from build123d import *

# Parameters (mm, degrees)
SKETCH1_R                = 1.75
BOSS_EXTRUDE1_DEPTH      = 23
FILLET3_R                = 10
BOSS_EXTRUDE2_DEPTH      = 4.5
BOSS_EXTRUDE2_DEPTH_BACK = 4
SKETCH3_R                = 1.75
SKETCH4_R                = 11.25
CUT_EXTRUDE1_DEPTH       = 7
SKETCH5_R                = 13
CUT_EXTRUDE2_DEPTH       = 1.5
SKETCH6_R                = 3
CUT_EXTRUDE3_DEPTH       = 12
CUT_EXTRUDE4_DEPTH       = 1
FILLET7_R                = 3
FILLET8_R                = 10


with BuildPart() as part:
    # Sketch1 → Boss-Extrude1 (new body)
    with BuildSketch(Plane.XY):
        with BuildLine():
            Line((-8.845360825, 11.520618557), (-14.845360825, 2.520618557))
            Line((-14.845360825, 2.520618557), (-14.845360825, -0.479381443))
            Line((-14.845360825, -0.479381443), (-9.845360825, -0.479381443))
            Line((-9.845360825, -0.479381443), (-8.845360825, 0.520618557))
            ThreePointArc((-8.845360825, 0.520618557), (-1.696742799, 7.320595709), (6.83903909, 12.26861112))
            Line((6.83903909, 12.26861112), (9.318301605, 19.26861112))
            ThreePointArc((9.318301605, 19.26861112), (-0.918731235, 18.102760488), (-8.845360825, 11.520618557))
        make_face()
        with Locations((-8.845360825, 5.020618557)):
            Circle(SKETCH1_R, mode=Mode.SUBTRACT)
        with Locations((3.154639175, 15.020618557)):
            Circle(SKETCH1_R, mode=Mode.SUBTRACT)
    extrude(amount=BOSS_EXTRUDE1_DEPTH)

    # Fillet3
    # the kernel refuses this fillet: 10 mm, written as the material it takes off along each edge
    with BuildSketch(Plane(origin=(-9.845360825, -0.479381443, -10.932362995), x_dir=(-1, 0, 0), z_dir=(0, 0, 1))) as fillet3_piece_1:
        with BuildLine():
            CenterArc((4.372945198, -10), FILLET3_R, 90, 46.455884642)
            Line((-2.87549632, -3.110871204), (-3.600340471, -2.421958325))
            ThreePointArc((-3.600340471, -2.421958325), (-1.769425443, -0.361263367), (-0.707106781, 0.707106781))
            Line((-0.707106781, 0.707106781), (0, 1))
            Line((0, 1), (4.372945198, 1))
            Line((4.372945198, 1), (4.372945198, 0))
        make_face()
    extrude(amount=44.86472599, mode=Mode.SUBTRACT)

    # Sketch3 → Boss-Extrude2 (add, two sides: drawn at the far end of the back side and taken through both)
    with BuildSketch(Plane.XY.offset(23).offset(-BOSS_EXTRUDE2_DEPTH_BACK)):
        with BuildLine():
            Line((-14.845360825, 2.520618557), (-14.845360825, -0.479381443))
            Line((-14.845360825, -0.479381443), (-12.565000182, -16.009144975))
            ThreePointArc((-12.565000182, -16.009144975), (8.709502938, -29.945300767), (20.013420995, -7.162799635))
            Line((20.013420995, -7.162799635), (9.318301605, 19.26861112))
            ThreePointArc((9.318301605, 19.26861112), (-0.918731235, 18.102760488), (-8.845360825, 11.520618557))
            Line((-8.845360825, 11.520618557), (-14.845360825, 2.520618557))
        make_face()
        with Locations((3.154639175, 15.020618557)):
            Circle(SKETCH3_R, mode=Mode.SUBTRACT)
        with Locations((-8.845360825, 5.020618557)):
            Circle(SKETCH3_R, mode=Mode.SUBTRACT)
    extrude(amount=BOSS_EXTRUDE2_DEPTH + BOSS_EXTRUDE2_DEPTH_BACK)

    # Sketch4 → Cut-Extrude1 (cut)
    with BuildSketch(Plane(origin=(0, 0, 19), x_dir=(-1, 0, 0), z_dir=(0, 0, -1))):
        with Locations((-4.254639175, -13.539381443)):
            Circle(SKETCH4_R)
    extrude(amount=-CUT_EXTRUDE1_DEPTH, mode=Mode.SUBTRACT)

    # Sketch5 → Cut-Extrude2 (cut)
    with BuildSketch(Plane(origin=(0, 0, 19), x_dir=(-1, 0, 0), z_dir=(0, 0, -1))):
        with Locations((-4.254639175, -13.539381443)):
            Circle(SKETCH5_R)
    extrude(amount=-CUT_EXTRUDE2_DEPTH, mode=Mode.SUBTRACT)

    # Sketch6 → Cut-Extrude3 (cut)
    with BuildSketch(Plane.XY.offset(27.5)):
        with Locations((-8.845360825, 5.020618557)):
            Circle(SKETCH6_R)
        with Locations((3.154639175, 15.020618557)):
            Circle(SKETCH6_R)
    extrude(amount=-CUT_EXTRUDE3_DEPTH, mode=Mode.SUBTRACT)

    # Sketch7 → Cut-Extrude4 (cut)
    with BuildSketch(Plane(origin=(0, 0, 19), x_dir=(-1, 0, 0), z_dir=(0, 0, -1))):
        with BuildLine():
            Line((-19.320512006, -15.73138888), (-26.521187379, 19.26861112))
            Line((-26.521187379, 19.26861112), (-9.318301605, 19.26861112))
            Line((-9.318301605, 19.26861112), (-6.83903909, 12.26861112))
            ThreePointArc((-6.83903909, 12.26861112), (0.552528201, 8.148031782), (6.969864505, 2.631489761))
            Line((6.969864505, 2.631489761), (-2.943055137, 1.26861112))
            ThreePointArc((-2.943055137, 1.26861112), (-15.267616881, -3.247010549), (-19.320512006, -15.73138888))
        make_face()
    extrude(amount=-CUT_EXTRUDE4_DEPTH, mode=Mode.SUBTRACT)

    # Fillet7
    # the kernel refuses this fillet: 3 mm, written as the material it takes off along each edge
    with BuildSketch(Plane(origin=(-8.845360825, 11.520618557, 27.5), x_dir=(0, 0, -1), z_dir=(-0.554700196225229, -0.8320502943378438, 0))) as fillet7_piece_1:
        with BuildLine():
            CenterArc((FILLET7_R, FILLET7_R), FILLET7_R, 180, 90)
            Line((0, FILLET7_R), (0, 0))
            Line((0, 0), (FILLET7_R, 0))
        make_face()
    extrude(amount=18.316653826, mode=Mode.SUBTRACT)
    with BuildSketch(Plane(origin=(-18.114165499, 21.781905941, 27.5), x_dir=(0, 0, -1), z_dir=(0.14528020772302286, -0.9893905504116943, 0))) as fillet7_piece_2:
        with BuildLine():
            CenterArc((FILLET7_R, FILLET7_R), FILLET7_R, 180, 90)
            Line((0, FILLET7_R), (0, 0))
            Line((0, 0), (FILLET7_R, 0))
        make_face()
    extrude(amount=38.196292556, mode=Mode.SUBTRACT)
    with BuildSketch(Plane(origin=(4.254639175, -13.539381443, 27.5), x_dir=(-0.9893905504116943, -0.14528020772302197, 0), z_dir=(-0.14528020772302197, 0.9893905504116943, 0))) as fillet7_piece_3:
        with BuildLine():
            CenterArc((17 - FILLET7_R, -FILLET7_R), FILLET7_R, 0, 90)
            Line((17 - FILLET7_R, 0), (17, 0))
            Line((17, 0), (17, -FILLET7_R))
        make_face()
    revolve(axis=Axis((4.254639175, -13.539381443, 27.5), (0, 0, 1)), revolution_arc=193.67655813, mode=Mode.SUBTRACT)
    with BuildSketch(Plane(origin=(6.154639175, 1.520618557, 27.5), x_dir=(0.5584515746383966, 0.8295371232102247, 0), z_dir=(0.8295371232102247, -0.5584515746383966, 0))) as fillet7_piece_4:
        with BuildLine():
            CenterArc((18.027756377 - FILLET7_R, -FILLET7_R), FILLET7_R, 0, 90)
            Line((18.027756377 - FILLET7_R, 0), (18.027756377, 0))
            Line((18.027756377, 0), (18.027756377, -FILLET7_R))
        make_face()
    revolve(axis=Axis((6.154639175, 1.520618557, 27.5), (0, 0, 1)), revolution_arc=90.258713785, mode=Mode.SUBTRACT)
    with BuildSketch(Plane(origin=(20.013420995, -7.162799635, 27.5), x_dir=(-0.9269871658598542, -0.3750930475643543, 0), z_dir=(-0.37509304756435435, 0.9269871658598543, 0))) as fillet7_piece_5:
        with BuildLine():
            CenterArc((FILLET7_R, -FILLET7_R), FILLET7_R, 90, 90)
            Line((0, -FILLET7_R), (0, 0))
            Line((0, 0), (FILLET7_R, 0))
        make_face()
    extrude(amount=36.013243471, mode=Mode.SUBTRACT)

    # Fillet8
    fillet8_edges = [part.edges().sort_by_distance(p)[0] for p in [
        (6.83903909, 12.26861112, 10),
    ]]
    fillet(fillet8_edges, radius=FILLET8_R)


solid = part.part
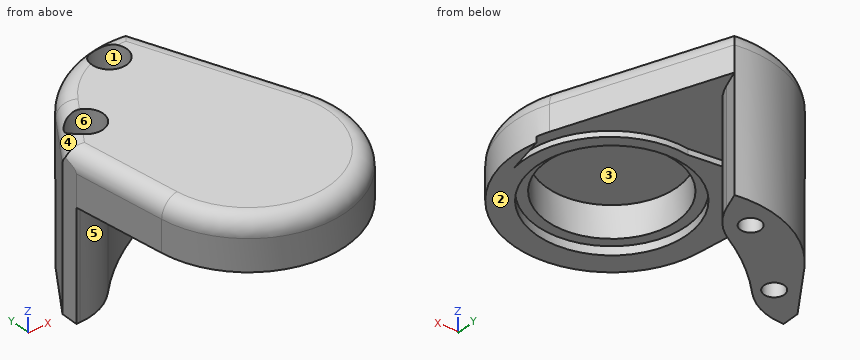
Input: part model. Units: mm. Frame: model coordinates. Face numbers are marked on the shaded views. A direction names the side the tool comes from. Give positions to 0.01 mm unless a question says otherwise; leave off trailing zeros. Write each loop counter-clockwise with the first axis right and the second up, starting at its lowest first coordinate (ties: lowest second). Pieces come first, ordered by that corner, then holes. Notation, with made-up numbers: M -6.5,79 L 31.5,79 A38 ccw 31.5,118 Z; hole C 15,-33.75 d3. An arc over 180 degrees is marked long. Write item = value, one per line. Start each with the question number.
1) First-contact query: pin 1 Ø1.8 at (x, y) = (-9, 4) entering from +Z; pin 2 Ø6 at (x, z) = (14.5, 23) entering from +Y; pin 3 Ø12 at (y, z) = (-22.5, 19.5) entering from -X; pin 4 Ø2 at (x, y) = (-8.85, 5.02) entering from +Z. Flat tips, straight axial feed; report the tip coordinate or a pass-through.
2) Cut plane A-A on z = 6.75. Return the cut outline in (x, y).
3) Material intervals for line 1 along Z through (x, y) = (9.5, -25); line 2 along Y through (x, z) = (-7.5, 21); line 3 along Y through (x, z) = (-4.5, 21.25), sorted ascending. Write a range as [from, to].
4) Reachability of the marked faces 1, 2 and 3 from +Z, -Z, +X, -X, +Y, -Y: full face, straight path, thin tool, end or side. Return the list, or none.
5) Draft query along Y for the marked faces 4, 5 and 6. Return one class per face: +Y half, -Y half, draft (parallel to the pull), parting line (faces both ways), or undercut.
6) Cut plane B-B on z = 16.5. Return the cut outline in (x, y).
Solved:
q1.pin_1 = 15.5
q1.pin_2 = 13.88
q1.pin_3 = -12.49
q1.pin_4 = through
q2.outline = M -14.85,-0.48 L -14.22,-0.48 A10 ccw -6.97,2.63 A42.07 cw 3.53,10.66 A10 ccw 8.2,16.12 L 9.32,19.27 A18.03 ccw -8.85,11.52 L -14.85,2.52 Z; hole C -8.85,5.02 d3.5; hole C 3.15,15.02 d3.5
q3.line_1 = [20.5, 27.5]
q3.line_2 = [-25.82, 2.34], [7.7, 13.29]
q3.line_3 = [-28.11, -20.6], [-6.47, 16.06]
q4.face_1 = +Z
q4.face_2 = -Z, +X, -Y
q4.face_3 = -Z
q5.face_4 = +Y half
q5.face_5 = -Y half
q5.face_6 = undercut
q6.outline = M -14.85,-0.48 L -14.22,-0.48 A10 ccw -6.97,2.63 A42.07 cw 3.53,10.66 A10 ccw 8.2,16.12 L 9.32,19.27 A18.03 ccw -8.85,11.52 L -14.85,2.52 Z; hole C -8.85,5.02 d6; hole C 3.15,15.02 d6
